The model under review builds one solid part; all positions refer to its coordinate system, in mm. Round coordinates to 2 decimals unless told otherwise and drop trailing zeros. Order: outer loops, then holes, each group sorted by start corner. A loop starts at its lowest first (then second) coordinate and runs counter-clockwise, first axis right, second up.
1) Mouldability with a two-part tool opening along Z and no side actions: class faces 1 (the face through (-16, 0.3, 37.5)), 2 (the face through (0, 9, 44)), 3 (the face through (-15.5, 0.3, 5.1)), 4 (the face through (25, 0, 22)) as pulls with the +Z half, pulls with the -Z half, needs draft (parallel to the pull), parting line crosses it, or undercut.
2) Consider section B-B (y = 0). Give the boundary of the cut face in (x, z).
3) Consider section A-A (z = 5). Give the boundary of the cut face in (x, y).
4) Consider section C-C (x = 0). Give the boundary of the cut face in (y, z).
5) To check wall thickness, follow L1, parallel to Z at x = -18, y = 9.5; L2, parallel to Y at x = 0, z = 24.5; L3, parallel to Z at x = 19, y = -3. State the ranges of each line that lie inside material, in increasing order.
6) Consider section D-D (x = -18). Give the boundary of the cut face in (y, z).
from build123d import *

# Parameters (mm, degrees)
F0_W     = 50
F0_H     = 38.5
F0_R     = 8
F1_DEPTH = 44
F2_R     = 2.5
F3_DEPTH = 38.5


with BuildPart() as f1:
    # F0 (on Top) → F1 (new body)
    with BuildSketch(Plane.XY):
        Rectangle(F0_W, F0_H)
        Circle(F0_R, mode=Mode.SUBTRACT)
    extrude(amount=F1_DEPTH)

    # F2 (on face) → F3 (cut)
    with BuildSketch(Plane(origin=(0, 19.25, 0), x_dir=(-1, 0, 0), z_dir=(0, 1, 0))):
        with Locations((18, 39)):
            Circle(F2_R)
        with Locations((18, 5)):
            Circle(F2_R)
        with Locations((-18, 39)):
            Circle(F2_R)
        with Locations((-18, 5)):
            Circle(F2_R)
    extrude(amount=-F3_DEPTH, mode=Mode.SUBTRACT)


solid = f1.part
Answer below:
1. face 1: undercut
1. face 2: pulls with the +Z half
1. face 3: undercut
1. face 4: needs draft
2. outline: (-25, 0) - (-8, 0) - (-8, 44) - (-25, 44) - close; (8, 0) - (25, 0) - (25, 44) - (8, 44) - close; hole circle Ø5 at (-18, 5); hole circle Ø5 at (-18, 39); hole circle Ø5 at (18, 5); hole circle Ø5 at (18, 39)
3. outline: (-25, -19.25) - (-20.5, -19.25) - (-20.5, 19.25) - (-25, 19.25) - close; (-15.5, -19.25) - (15.5, -19.25) - (15.5, 19.25) - (-15.5, 19.25) - close; (20.5, -19.25) - (25, -19.25) - (25, 19.25) - (20.5, 19.25) - close; hole circle Ø16 at (0, 0)
4. outline: (-19.25, 0) - (-8, 0) - (-8, 44) - (-19.25, 44) - close; (8, 0) - (19.25, 0) - (19.25, 44) - (8, 44) - close
5. L1: z = 0 to 2.5, 7.5 to 36.5, 41.5 to 44
5. L2: y = -19.25 to -8, 8 to 19.25
5. L3: z = 0 to 2.71, 7.29 to 36.71, 41.29 to 44
6. outline: (-19.25, 0) - (19.25, 0) - (19.25, 2.5) - (-19.25, 2.5) - close; (-19.25, 7.5) - (19.25, 7.5) - (19.25, 36.5) - (-19.25, 36.5) - close; (-19.25, 41.5) - (19.25, 41.5) - (19.25, 44) - (-19.25, 44) - close
